from build123d import *

# Parameters (mm, degrees)
SKETCH_W        = 83.7
SKETCH_H        = 24
SKETCH_R        = 2
PAD_DEPTH       = 5
SKETCH001_W     = 11.4
SKETCH001_H     = 11.4
POCKET_DEPTH    = 5.001
SKETCH002_W     = 5
SKETCH002_H     = 11.4
PAD001_DEPTH    = 25
SKETCH003_R     = 1.5
POCKET001_DEPTH = 74.701


with BuildPart() as part:
    # Sketch → Pad (new body)
    with BuildSketch(Plane.XY):
        with Locations((41.85, 12)):
            Rectangle(SKETCH_W, SKETCH_H)
        with Locations((33.48, 7)):
            Circle(SKETCH_R, mode=Mode.SUBTRACT)
        with Locations((16.74, 7)):
            Circle(SKETCH_R, mode=Mode.SUBTRACT)
        with Locations((50.22, 7)):
            Circle(SKETCH_R, mode=Mode.SUBTRACT)
        with Locations((66.96, 7)):
            Circle(SKETCH_R, mode=Mode.SUBTRACT)
    extrude(amount=PAD_DEPTH)

    # Sketch001 → Pocket (cut, through all)
    with BuildSketch(Plane.XY.offset(5)):
        with Locations((64, 18.3)):
            Rectangle(SKETCH001_W, SKETCH001_H)
        with Locations((19.7, 18.3)):
            Rectangle(SKETCH001_W, SKETCH001_H)
    extrude(amount=-POCKET_DEPTH, mode=Mode.SUBTRACT)

    # Sketch002 → Pad001 (new body)
    with BuildSketch(Plane.XY.offset(5)):
        with Locations((11.5, 18.3)):
            Rectangle(SKETCH002_W, SKETCH002_H)
        with Locations((27.9, 18.3)):
            Rectangle(SKETCH002_W, SKETCH002_H)
        with Locations((55.8, 18.3)):
            Rectangle(SKETCH002_W, SKETCH002_H)
        with Locations((72.2, 18.3)):
            Rectangle(SKETCH002_W, SKETCH002_H)
    extrude(amount=PAD001_DEPTH)

    # Sketch003 → Pocket001 (cut, through all)
    with BuildSketch(Plane.YZ.offset(74.7)):
        with Locations((18.179388, 19)):
            Circle(SKETCH003_R)
        with Locations((18.179388, 11)):
            Circle(SKETCH003_R)
    extrude(amount=-POCKET001_DEPTH, mode=Mode.SUBTRACT)


solid = part.part
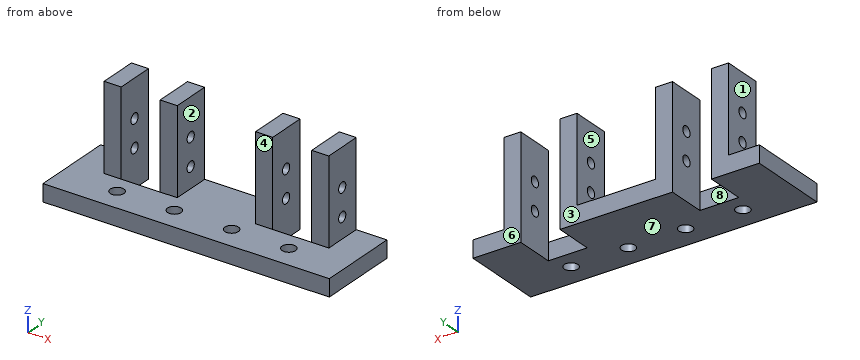
Can you work these out from the model? Positions are in its coordinate system, mm. Face numbers are marked on the shaded views. A direction names the side the tool comes from. Round coordinates to 2 decimals unless told otherwise and drop trailing zeros. Write each loop counter-clockwise with the first axis right and the second up, starting at its lowest first coordinate (ties: lowest second). Pieces come first, ordered by that corner, then holes. Notation, with made-up numbers: (74.25, 25.5) -> (85.25, 25.5) arc R12 cw to (85.25, 34.5) -> close; hole circle Ø7 at (57, 83). An arc over 180 degrees is marked (long way). One line per question, with ' | ' between items. Start each with the question number.
1) Suppose I cut it at C-C on x = 16.74. Write out the boundary of the cut face in (y, z), then the cut area to 3 significant figures.
2) On a 3-axis mill with a long thin cutter (end or side, diameter ignored), from which of +Z, -Z, +X, -X, +Y, -Y can I reach the whole of each face in a straight line? I mean the marked faces 4, 5, 6, 7 and 8. Say none if no direction works.
3) Suppose I cut it at B-B on y = 20.5. Write out the boundary of the cut face in (x, z).
4) Suppose I cut it at A-A on z = 25. Write out the boundary of the cut face in (x, y), then the cut area to 3 significant figures.
5) I'm going to push flat-ended pins straight in: P1, Ø2, axis at y = 17.5, z = 12.5, coming from the -X side; P2, Ø4, axis at x = 55, z = 12.5, coming from the -Y side; P3, Ø6, axis at y = 19, z = 16.5, coming from the +X side; P4, Ø12.5, axis at y = 16, z = 7.5, coming from the -X side. Where does each tip first touch, or does it pass through?
6) I need wall thicknesses on line 1 (X direction, y = 20.25, z = 21.75); line 2 (X direction, y = 15.5, z = 4); line 3 (Y direction, x = 50.22, z = 1.6). Which ranges of each line are inside material? Lowest first, please. Write a range as [from, to].
7) If we mould it in two halves opening along X, with no side actions, what happens to the marked faces 1, 2 and 3? For each: released by +X, released by -X, zero draft, split by the parting line, or undercut.
8) Suppose I cut it at D-D on z = 11. Count the separate pieces of the cut face and the enclosed holes in it, then the cut area to 3 significant figures.
Return value:
1) outline: (0, 0) -> (5, 0) -> (5, 5) -> (0, 5) -> close; (9, 0) -> (12.6, 0) -> (12.6, 5) -> (9, 5) -> close | area: 43.0 mm2
2) face 4: +Z, +X, -X, -Y | face 5: +Z, +Y, -Y | face 6: +Z, -Z, +X, -X, +Y | face 7: -Z, +X, -X, +Y, -Y | face 8: +Z, -Z, +Y
3) outline: (0, 0) -> (14, 0) -> (14, 30) -> (9, 30) -> (9, 5) -> (0, 5) -> close; (25.4, 0) -> (58.3, 0) -> (58.3, 30) -> (53.3, 30) -> (53.3, 5) -> (30.4, 5) -> (30.4, 30) -> (25.4, 30) -> close; (69.7, 0) -> (83.7, 0) -> (83.7, 5) -> (74.7, 5) -> (74.7, 30) -> (69.7, 30) -> close
4) outline: (9, 12.6) -> (14, 12.6) -> (14, 24) -> (9, 24) -> close; (25.4, 12.6) -> (30.4, 12.6) -> (30.4, 24) -> (25.4, 24) -> close; (53.3, 12.6) -> (58.3, 12.6) -> (58.3, 24) -> (53.3, 24) -> close; (69.7, 12.6) -> (74.7, 12.6) -> (74.7, 24) -> (69.7, 24) -> close | area: 228 mm2
5) P1: stops at x = 9 | P2: stops at y = 12.6 | P3: stops at x = 74.7 | P4: stops at x = 0
6) line 1: x = [9, 14], [25.4, 30.4], [53.3, 58.3], [69.7, 74.7] | line 2: x = [0, 14], [25.4, 58.3], [69.7, 83.7] | line 3: y = [0, 5], [9, 24]
7) face 1: released by -X | face 2: undercut | face 3: zero draft
8) separate pieces: 8 | enclosed holes: 0 | area: 168 mm2
